Autodesk Fusion 360 part; units mm, degrees
sketch "Sketch1" plane through (0, 0, 0) normal (0, 0, 1) x (1, 0, 0)
  circle A0 centre (0, 0) radius 8
  circle A1 centre (0, 0) radius 4
  dimension "d1" = 8
  dimension "d2" = 16
extrude "Extrude1" add sketch "Sketch1" along normal blind 25 makes body 1
fillet "Fillet1" radius 0.2 2 edges at (-3.7293, 1.4465, 25) (-3.7293, 1.4465, 0) on bodies 1
fillet "Fillet2" radius 0.4 2 edges at (-7.4586, -2.8929, 25) (-7.4586, -2.8929, 0) on bodies 1
copy_body "Body->Comp1" bodies 1 removing the originals makes body 2 in component "Component"
component "Component" placed x (1, 0, 0) y (0, 1, 0) z (0, 0, 1) at (0, 0, 0)
Verification items for the finished model (mm, model axes). Give positions to 0.01 mm unless a question says otherwise; leave off trailing zeros. Loops run counter-clockwise (first coordinate to the right, second up) from the corner with the lowest first, then second, coordinate; pieces in that order, holes last.
1. Section check C-C, the plane z = 18.5. Enter the section's corners in (x, y).
2. Go/stop test with flat-tipped pins: pin 1 Ø6 at (y, z) = (-3.5, 15.5) entering from -X; pin 2 Ø1.5 at (x, z) = (3.5, 4) entering from +Y; pin 3 Ø5 at (y, z) = (5, 11.5) entering from +X; pin 4 Ø1.5 at (x, y) = (3.5, -0.5) entering from +Z. Record where each tip stops, or that it passes through.
3. Section check A-A, the plane y = 0. Enter the section's corners in (x, z), then the cut area to 3 significant figures.
4. Mould release check, pull along Y, two halves, no side actions. Record for faces 1 (the cylindrical face through (-1.73, 7.81, 12.33)), 2 (the flat face through (3.3, -3.3, 25)), 3 (the cylindrical face through (-0.867, 3.905, 12.328)): released by +Y, released by -Y, zero draft, split by the parting line, or undercut.
5. Thickness scan on line 1 (Y direction, x = 0, z = 19); line 2 (X direction, y = -2, z = 19.25); line 3 (X direction, y = 0.25, z = 4). Record the ranges inside material, lowest first.
Geometry says:
1. outline: circle Ø16 at (0, 0); hole circle Ø8 at (0, 0)
2. pin 1: stops at x = -7.98
2. pin 2: stops at y = 7.51
2. pin 3: stops at x = 7.6
2. pin 4: stops at z = 25
3. outline: (-8, 0.4) arc R0.4 ccw to (-7.6, 0) - (-4.2, 0) arc R0.2 ccw to (-4, 0.2) - (-4, 24.8) arc R0.2 ccw to (-4.2, 25) - (-7.6, 25) arc R0.4 ccw to (-8, 24.6) - close; (4, 0.2) arc R0.2 ccw to (4.2, 0) - (7.6, 0) arc R0.4 ccw to (8, 0.4) - (8, 24.6) arc R0.4 ccw to (7.6, 25) - (4.2, 25) arc R0.2 ccw to (4, 24.8) - close
3. area: 200 mm2
4. face 1: split by the parting line
4. face 2: zero draft
4. face 3: undercut
5. line 1: y = -8 to -4, 4 to 8
5. line 2: x = -7.75 to -3.46, 3.46 to 7.75
5. line 3: x = -8 to -3.99, 3.99 to 8
